Solid Edge part; units mm, degrees
sketch "Sketch1" plane through (0, 0, 0) normal (0, -1, 0) x (1, 0, 0)
  line L0 (-4.1692, 30) -> (22.4208, 30)
  line L1 (22.4208, 30) -> (35.8285, 20.6779)
  line L2 (35.8285, 20.6779) -> (35.8285, -12.6896)
  line L3 (35.8285, -12.6896) -> (32.1463, -15.8179)
  line L4 (32.1463, -15.8179) -> (5.0763, -15.8179)
  line L5 (5.0763, -15.8179) -> (-17.825, 4.6726)
  line L6 (-17.825, 4.6726) -> (-17.825, 22.1126)
  line L7 (-17.825, 22.1126) -> (-4.1692, 30)
  dimension "D1" = 4.1692
  dimension "D2" = 17.825
  dimension "D3" = 32.1463
  dimension "D4" = 22.4208
  dimension "D5" = 35.8285
  dimension "D6" = 35.8285
extrude "Protrusion1" add sketch "Sketch1" against normal blind 3
properties part number "049" material "Acryl, hochfest"
For this review, take the finished solid that the model builds, in its own axes (mm). Coordinates: 2 decimals unless noted, no trailing zeros. Order: outer loops, then holes, each group sorted by start corner. A loop starts at its lowest first (then second) coordinate and runs counter-clockwise, first axis right, second up. Notation, with made-up numbers: (71.5, -20.5) - (76.5, -20.5) arc R28 cw to (76.5, 18.5) - close; hole circle Ø2 at (56, 76). An arc over 180 degrees is marked (long way). Answer as CSV lines item,"result". Start each with the question number.
1) To check wall thickness, follow line 1 along Z through (x, y) = (-13, 0.75); line 2 along X through (y, z) = (1.6, -11); line 3 along X through (y, z) = (2.85, 26.5). State the ranges of each line that lie inside material, in increasing order. Write a range as [from, to].
2) Add section C-C (z = -4). State the section outline as (x, y) points.
3) Add section A-A (y = 1.65). State the section outline as (x, z) points (1 decimal), then the cut area to 3 significant figures.
4) Add section B-B (x = -2). State the section outline as (y, z) points.
Result:
1,line 1,"[0.36, 24.9]"
1,line 2,"[-0.31, 35.83]"
1,line 3,"[-10.23, 27.45]"
2,outline,"(-8.13, 0) - (35.83, 0) - (35.83, 3) - (-8.13, 3) - close"
3,outline,"(-17.8, 4.7) - (5.1, -15.8) - (32.1, -15.8) - (35.8, -12.7) - (35.8, 20.7) - (22.4, 30) - (-4.2, 30) - (-17.8, 22.1) - close"
3,area,"2,100 mm^2"
4,outline,"(0, -9.49) - (3, -9.49) - (3, 30) - (0, 30) - close"
